The listing builds one solid part. Answer for the finished solid, in the listing's coordinates (mm). Round coordinates to 2 decimals unless told otherwise and drop trailing zeros. Write each loop counter-clockwise with the first axis right and the second up, starting at its lowest first coordinate (ties: lowest second). Pieces come first, ordered by that corner, then holes. Notation, with made-up numbers: (21, -24) - (58, -24) arc R25 cw to (58, 10) - close; hole circle Ø1 at (25, -4.75). An arc over 180 degrees is marked (long way). Return JSON: item names as keys, results as strings. Group by question number.
from build123d import *

# Parameters (mm, degrees)
F0_W     = 19.9
F0_H     = 22.1
F1_DEPTH = 1.7
F2_D     = 3.1
F2_DEPTH = 5
F3_D     = 1
F3_DEPTH = 5
F4_R     = 8.2
F5_DEPTH = 13.8
F6_R     = 1.5


with BuildPart() as f1:
    # F0 (on Top) → F1 (new body)
    with BuildSketch(Plane.XY):
        Rectangle(F0_W, F0_H)
    extrude(amount=-F1_DEPTH)

    # F2
    with Locations(Plane.XY):
        with Locations((-5.19, 8.49), (7.41, -8.51)):
            Hole(F2_D / 2, depth=F2_DEPTH)

    # F3
    with Locations(Plane.XY):
        with Locations((-8.75, 5.89), (-8.75, 3.35), (-8.75, 0.81), (-8.75, -1.73), (-8.75, -4.27), (-8.75, -6.81), (-8.75, -9.35)):
            Hole(F3_D / 2, depth=F3_DEPTH)

    # F4 (on face) → F5 (join)
    with BuildSketch(Plane(origin=(0, 0, -1.7), x_dir=(1, 0, 0), z_dir=(0, 0, -1))):
        Circle(F4_R)
    extrude(amount=F5_DEPTH)

    # F6
    f6_edges = [f1.edges().sort_by_distance(p)[0] for p in [
        (-8.2, 0, -15.5),
    ]]
    fillet(f6_edges, radius=F6_R)


solid = f1.part
(1) Find section C-C (y = 0). Write down the section's boundary in (x, z), plus the area to 3 significant figures.
(2) Determine the mould class of faces 1 (the flat face through (4, 8, -1.7)), 2 (the cylindrical face through (-1.07, -8.13, -7.76)), 3 (the cylindrical face through (-9.212, -9.542, -0.862)) for opening direction Y: +Y half, -Y half, draft (parallel to the pull), parting line (faces both ways), or undercut.
(3) Consider line 1 (Y direction, x = -5.19, z = -0.4); line 2 (X direction, y = -0.25, z = -4); line 3 (Y direction, x = 7.41, z = -0.45). Determine where each line is inside the solid, lowest interval first.
(4) Find section A-A (y = -8.51). Write down the section's boundary in (x, z), plus the area to 3 significant figures.
(5) Find section D-D (z = -10.75). Write down the section's boundary in (x, y), plus the area to 3 significant figures.
(6) Flat-ended cylindrical pins translate along their axes: pin 1 (1.5 mm diameter, centred on x = 4.5, z = -6.5, fed in from -Y); pin 2 (8 mm diameter, centred on y = -7.5, z = -9, fed in from +X); pin 3 (3 mm diameter, centred on y = 0.5, z = -10.5, fed in from -X). Find the tip coordinate at first contact, or state that the pin passes through.
(7) Find section B-B (x = 0). Write down the section's boundary in (y, z).
Check sheet entries:
{
 "1": {"outline": "(-9.95, -1.7) - (-8.2, -1.7) - (-8.2, -14) arc R1.5 ccw to (-6.7, -15.5) - (6.7, -15.5) arc R1.5 ccw to (8.2, -14) - (8.2, -1.7) - (9.95, -1.7) - (9.95, 0) - (-9.95, 0) - close", "area": "259 mm^2"},
 "2": {"face 1": "draft", "face 2": "parting line", "face 3": "undercut"},
 "3": {"line 1": "y = -11.05 to 6.94, 10.04 to 11.05", "line 2": "x = -8.2 to 8.2", "line 3": "y = -11.05 to -10.06, -6.96 to 11.05"},
 "4": {"outline": "(-9.95, -1.7) - (5.86, -1.7) - (5.86, 0) - (-9.95, 0) - close; (8.96, -1.7) - (9.95, -1.7) - (9.95, 0) - (8.96, 0) - close", "area": "28.6 mm^2"},
 "5": {"outline": "circle Ø16.4 at (0, 0)", "area": "211 mm^2"},
 "6": {"pin 1": "stops at y = -7.29", "pin 2": "stops at x = 7.42", "pin 3": "stops at x = -8.2"},
 "7": {"outline": "(-11.05, -1.7) - (-8.2, -1.7) - (-8.2, -14) arc R1.5 ccw to (-6.7, -15.5) - (6.7, -15.5) arc R1.5 ccw to (8.2, -14) - (8.2, -1.7) - (11.05, -1.7) - (11.05, 0) - (-11.05, 0) - close"}
}
